Work out the finished part from the listing and answer in its coordinate system (mm). Face numbers are marked on the shaded views. A direction names the side the tool comes from. Round coordinates to 2 decimals unless told otherwise and drop trailing zeros. Write each loop counter-clockwise with the first axis right and the second up, starting at its lowest first coordinate (ties: lowest second). Pieces come first, ordered by that corner, then holes. Notation, with made-up numbers: M 1.25,79.5 L 44.25,79.5 A23 ccw 44.25,96.5 Z; hole C 53.25,-32 d10. An arc over 180 degrees is marked long. Answer in a Markdown table with one row per item.
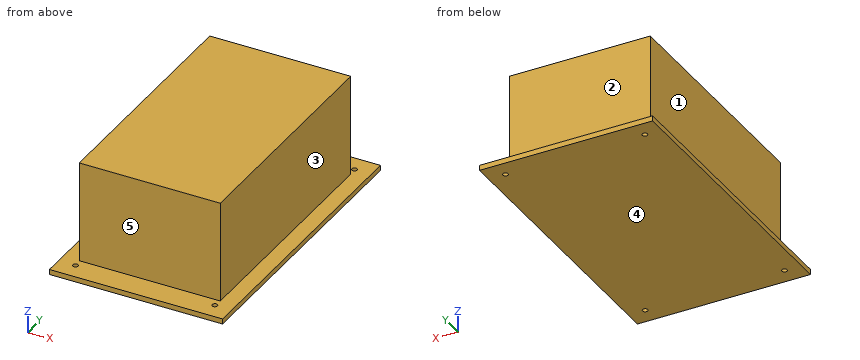
```python
from build123d import *

# Parameters (mm, degrees)
BOX_SKETCH_W              = 33.4
BOX_SKETCH_H              = 57
BOX_EXTRUDE_DEPTH         = 25.2
FLANGE_SKETCH_W           = 41
FLANGE_SKETCH_H           = 69
FLANGE_EXTRUDE_DEPTH      = 1.23456789
MOUNTHOLES_CUT_DEPTH      = 48.387129054
MOUNTHOLES_CUT_DEPTH_BACK = 48.387129054
MOUNTHOLES_SKETCH_R       = 0.617283945


with BuildPart() as part:
    # box_sketch → box_extrude (new body)
    with BuildSketch(Plane.XY):
        Rectangle(BOX_SKETCH_W, BOX_SKETCH_H)
    extrude(amount=BOX_EXTRUDE_DEPTH)

    # flange_sketch → flange_extrude (add)
    with BuildSketch(Plane.XY):
        Rectangle(FLANGE_SKETCH_W, FLANGE_SKETCH_H)
    extrude(amount=FLANGE_EXTRUDE_DEPTH)

    # mountHoles_sketch → mountHoles_cut (cut, two sides: drawn at the far end of the back side and taken through both)
    with BuildSketch(Plane.XY.offset(-MOUNTHOLES_CUT_DEPTH_BACK)):
        with Locations((16.5, -30.5)):
            Circle(MOUNTHOLES_SKETCH_R)
        with Locations((16.5, 30.5)):
            Circle(MOUNTHOLES_SKETCH_R)
        with Locations((-16.5, -30.5)):
            Circle(MOUNTHOLES_SKETCH_R)
        with Locations((-16.5, 30.5)):
            Circle(MOUNTHOLES_SKETCH_R)
    extrude(amount=MOUNTHOLES_CUT_DEPTH + MOUNTHOLES_CUT_DEPTH_BACK, mode=Mode.SUBTRACT)


solid = part.part
```
1. A tool of negligible diameter and unlimited length cuts with its end or side. For the marked faces 1, 2, 3, 4 and 5, from which of +Z, -Z, +X, -X, +Y, -Y can it reach the whole face along a straight path? Write none if from no direction.
Calculated:
| item | result |
|---|---|
| face 1 | +Z, -X, +Y, -Y |
| face 2 | +Z, +X, -X, +Y |
| face 3 | +Z, +X, +Y, -Y |
| face 4 | -Z, +X, -X, +Y, -Y |
| face 5 | +Z, +X, -X, -Y |
2. The part is cut by section A-A (y = -16). Determine the outline of the cut face in (x, z), plus the area to 3 significant figures.
Calculated:
| item | result |
|---|---|
| outline | M -20.5,0 L 20.5,0 L 20.5,1.23 L 16.7,1.23 L 16.7,25.2 L -16.7,25.2 L -16.7,1.23 L -20.5,1.23 Z |
| area | 851 mm² |
3. Given pin 1 (10 mm diameter, centred on x = 13, z = 8, fed in from -Y); pin 2 (1 mm diameter, centred on y = 1.5, z = 9.5, fed in from +X); pin 3 (10 mm diameter, centred on y = -10.5, z = 20.5, fed in from -X); pin 4 (1 mm diameter, centred on x = 16.5, y = -30.5, fed in from +Z), each flat-ended and moving along its own axis, determine where each tip first touches the part or whether it passes through.
Calculated:
| item | result |
|---|---|
| pin 1 | stops at y = -28.5 |
| pin 2 | stops at x = 16.7 |
| pin 3 | stops at x = -16.7 |
| pin 4 | passes through |
4. Consider line 1 along Y through (x, z) = (-16.5, 0.55); line 2 along X through (y, z) = (-30.5, 0.3); line 3 along Y through (x, z) = (5, 13.5). Determine where each line is inside the solid, lowest interval first. Write a range as from..to.
Calculated:
| item | result |
|---|---|
| line 1 | y = -34.5..-31.12, -29.88..29.88, 31.12..34.5 |
| line 2 | x = -20.5..-17.12, -15.88..15.88, 17.12..20.5 |
| line 3 | y = -28.5..28.5 |
5. The part is cut by section C-C (z = 9). Determine the outline of the cut face in (x, y), plus the area to 3 significant figures.
Calculated:
| item | result |
|---|---|
| outline | M -16.7,-28.5 L 16.7,-28.5 L 16.7,28.5 L -16.7,28.5 Z |
| area | 1,900 mm² |
6. The part is cut by section B-B (x = -15). Determine the outline of the cut face in (y, z).
Calculated:
| item | result |
|---|---|
| outline | M -34.5,0 L 34.5,0 L 34.5,1.23 L 28.5,1.23 L 28.5,25.2 L -28.5,25.2 L -28.5,1.23 L -34.5,1.23 Z |
